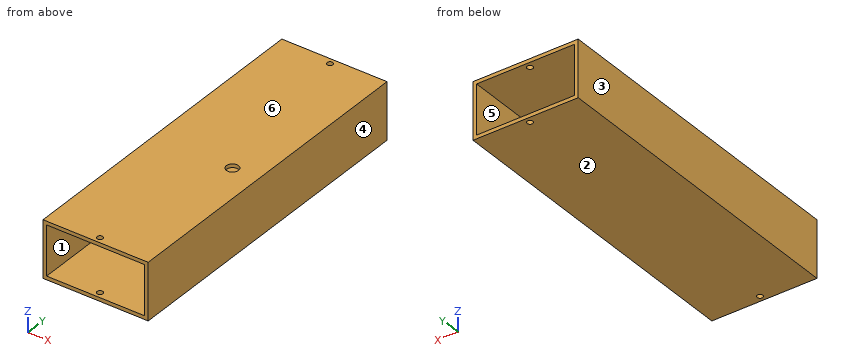
```python
from build123d import *

# Parameters (mm, degrees)
F0_W     = 43.5
F0_H     = 23.5
F0_W_2   = 40.5
F0_H_2   = 20.5
F1_DEPTH = 135
F2_R     = 2.5
F3_DEPTH = 1.5
F4_R     = 1.2
F5_DEPTH = 25


with BuildPart() as f1:
    # F0 (on Front) → F1 (new body)
    with BuildSketch(Plane.XZ):
        Rectangle(F0_W, F0_H)
        Rectangle(F0_W_2, F0_H_2, mode=Mode.SUBTRACT)
    extrude(amount=F1_DEPTH)

    # F2 (on face) → F3 (cut, through all)
    with BuildSketch(Plane.XY.offset(11.75)):
        with Locations((10.875, -72.5)):
            Circle(F2_R)
    extrude(amount=-F3_DEPTH, mode=Mode.SUBTRACT)

    # F4 (on face) → F5 (cut)
    with BuildSketch(Plane.XY.offset(11.75)):
        with Locations((0, -132.5)):
            Circle(F4_R)
        with Locations((0, -2.5)):
            Circle(F4_R)
    extrude(amount=-F5_DEPTH, mode=Mode.SUBTRACT)


solid = f1.part
```
Read the model definition and answer for the solid it produces. Units are mm, in the model's axes. Face numbers are marked on the shaded views. A direction names the side the tool comes from. Round coordinates to 2 decimals unless told otherwise and drop trailing zeros. Write each loop counter-clockwise with the first axis right and the second up, starting at its lowest first coordinate (ties: lowest second). Pieces come first, ordered by that corner, then holes. Notation, with made-up numbers: (85, 21.25) - (127, 21.25) arc R32 ccw to (127, 55.25) - close; hole circle Ø3 at (-35, 66.5). An arc over 180 degrees is marked (long way). One line per item, written item: value.
Q1. Which of the six approach directions +Z, -Z, +X, -X, +Y, -Y give full straight-line access (tool end or side, diameter ignored) to the marked faces 1 and 2?
The answers:
face 1: +Y, -Y
face 2: -Z, +X, -X, +Y, -Y
Q2. Find section A-A (y = -2.5). Determine the outline of the cut face in (x, z), and give its area (3 significant figures).
The answers:
outline: (-21.75, -11.75) - (-1.2, -11.75) - (-1.2, -10.25) - (-20.25, -10.25) - (-20.25, 10.25) - (-1.2, 10.25) - (-1.2, 11.75) - (-21.75, 11.75) - close; (1.2, -11.75) - (21.75, -11.75) - (21.75, 11.75) - (1.2, 11.75) - (1.2, 10.25) - (20.25, 10.25) - (20.25, -10.25) - (1.2, -10.25) - close
area: 185 mm2
Q3. Find section C-C (z = -8.5). Determine the outline of the cut face in (x, y), and give its area (3 significant figures).
The answers:
outline: (-21.75, -135) - (-20.25, -135) - (-20.25, 0) - (-21.75, 0) - close; (20.25, -135) - (21.75, -135) - (21.75, 0) - (20.25, 0) - close
area: 405 mm2
Q4. For a pull along X with two mould halves and no side action, classify the marked faces 3, 4, 5 and 6 as pulls with the +X half, pulls with the -X half, needs draft (parallel to the pull), parting line crosses it, or undercut.
The answers:
face 3: pulls with the -X half
face 4: pulls with the +X half
face 5: undercut
face 6: needs draft
Q5. Find section B-B (x = -16.5). Determine the outline of the cut face in (y, z), and give its area (3 significant figures).
The answers:
outline: (-135, -11.75) - (0, -11.75) - (0, -10.25) - (-135, -10.25) - close; (-135, 10.25) - (0, 10.25) - (0, 11.75) - (-135, 11.75) - close
area: 405 mm2
Q6. Find section D-D (x = 0). Determine the outline of the cut face in (y, z), and give its area (3 significant figures).
The answers:
outline: (-135, -11.75) - (-133.7, -11.75) - (-133.7, -10.25) - (-135, -10.25) - close; (-135, 10.25) - (-133.7, 10.25) - (-133.7, 11.75) - (-135, 11.75) - close; (-131.3, -11.75) - (-3.7, -11.75) - (-3.7, -10.25) - (-131.3, -10.25) - close; (-131.3, 10.25) - (-3.7, 10.25) - (-3.7, 11.75) - (-131.3, 11.75) - close; (-1.3, -11.75) - (0, -11.75) - (0, -10.25) - (-1.3, -10.25) - close; (-1.3, 10.25) - (0, 10.25) - (0, 11.75) - (-1.3, 11.75) - close
area: 391 mm2
Q7. Straight lines are drawn through the part: line 1 (Y direction, x = 0, z = -10.75); line 2 (X direction, y = -132.5, z = -11.35); line 3 (Z direction, x = 10.5, y = -58). For each, find the intervals that lie inside material, in ascending order. Write a range as from..to.
The answers:
line 1: y = -135..-133.7, -131.3..-3.7, -1.3..0
line 2: x = -21.75..-1.2, 1.2..21.75
line 3: z = -11.75..-10.25, 10.25..11.75
